```python
from build123d import *

# Parameters (mm, degrees)
BOSS_EXTRUDE1_DEPTH = 6.35
CUT_EXTRUDE18_DEPTH = 10
SKETCH20_R          = 57.15
BOSS_EXTRUDE5_DEPTH = 19.05
CUT_EXTRUDE14_DEPTH = 106.568863781
SKETCH22_R          = 3.175
CUT_EXTRUDE15_DEPTH = 112.672649781
SKETCH24_R          = 5
CUT_EXTRUDE16_DEPTH = 117.574618566
SKETCH25_R          = 2.38125
CUT_EXTRUDE17_DEPTH = 10
CHAMFER2_SIZE       = 2.5
FILLET1_R           = 1.5875
SKETCH28_R          = 30.48
CUT_EXTRUDE19_DEPTH = 105.22344993
CUT_EXTRUDE20_DEPTH = 100.947550226
CUT_EXTRUDE21_DEPTH = 94.849309593


with BuildPart() as part:
    # Sketch1 → Boss-Extrude1 (new body)
    with BuildSketch(Plane(origin=(0, 0, 0), x_dir=(0, 0, -1), z_dir=(1, 0, 0))):
        with BuildLine():
            Line((-30.369265969, -2.595782062), (-25.307721641, -61.813151718))
            ThreePointArc((-25.307721641, -61.813151718), (0, -85.05), (25.307721641, -61.813151718))
            Line((25.307721641, -61.813151718), (30.369265969, -2.595782062))
            ThreePointArc((30.369265969, -2.595782062), (0, 30.48), (-30.369265969, -2.595782062))
        make_face()
        Polygon((4.353205728, 11.960334439), (-11.960334439, 4.353205728), (-4.353205728, -11.960334439), (11.960334439, -4.353205728), align=None, mode=Mode.SUBTRACT)
    extrude(amount=BOSS_EXTRUDE1_DEPTH)

    # Sketch19 → Cut-Extrude18 (cut)
    with BuildSketch(Plane(origin=(6.35, 0, 0), x_dir=(0, 0, -1), z_dir=(1, 0, 0))):
        with BuildLine():
            Line((13.556349186, -39.093650814), (13.556349186, -44.093650814))
            ThreePointArc((13.556349186, -44.093650814), (15.556349186, -46.093650814), (17.556349186, -44.093650814))
            Line((17.556349186, -44.093650814), (17.556349186, -39.093650806))
            ThreePointArc((17.556349186, -39.093650806), (15.556349182, -37.093650814), (13.556349186, -39.093650814))
        make_face()
        with BuildLine():
            Line((-10, -54.65), (-10, -59.65))
            ThreePointArc((-10, -59.65), (0, -69.65), (10, -59.65))
            Line((10, -59.65), (10, -54.65))
            ThreePointArc((10, -54.65), (0, -44.65), (-10, -54.65))
        make_face()
        with BuildLine():
            Line((17.556349186, -75.206349194), (17.556349186, -70.206349186))
            ThreePointArc((17.556349186, -70.206349186), (15.556349186, -68.206349186), (13.556349186, -70.206349186))
            Line((13.556349186, -70.206349186), (13.556349186, -75.206349186))
            ThreePointArc((13.556349186, -75.206349186), (15.556349182, -77.206349186), (17.556349186, -75.206349194))
        make_face()
        with BuildLine():
            Line((-17.556349186, -39.093650806), (-17.556349186, -44.093650814))
            ThreePointArc((-17.556349186, -44.093650814), (-15.556349186, -46.093650814), (-13.556349186, -44.093650814))
            Line((-13.556349186, -44.093650814), (-13.556349186, -39.093650814))
            ThreePointArc((-13.556349186, -39.093650814), (-15.556349182, -37.093650814), (-17.556349186, -39.093650806))
        make_face()
        with BuildLine():
            Line((-13.556349186, -75.206349186), (-13.556349186, -70.206349186))
            ThreePointArc((-13.556349186, -70.206349186), (-15.556349186, -68.206349186), (-17.556349186, -70.206349186))
            Line((-17.556349186, -70.206349186), (-17.556349186, -75.206349194))
            ThreePointArc((-17.556349186, -75.206349194), (-15.556349182, -77.206349186), (-13.556349186, -75.206349186))
        make_face()
    extrude(amount=-CUT_EXTRUDE18_DEPTH, mode=Mode.SUBTRACT)

    # Sketch20 → Boss-Extrude5 (add)
    with BuildSketch(Plane(origin=(6.35, 0, 0), x_dir=(0, 0, -1), z_dir=(1, 0, 0))):
        with Locations(Location((0, 0, 0), (0, 0, 242.654471511))):
            Circle(SKETCH20_R)
    extrude(amount=BOSS_EXTRUDE5_DEPTH)

    # Sketch21 → Cut-Extrude14 (cut, through all)
    with BuildSketch(Plane.ZY):
        Polygon((-19.067760927, 15.897892729), (-24.435012851, 4.387783834), (-10.840396045, -1.951490092), (-5.473144121, 9.558618803), align=None)
        Polygon((-11.960334439, -4.353205728), (-4.353205728, 11.960334439), (11.960334439, 4.353205728), (4.353205728, -11.960334439), align=None)
        Polygon((10.840396045, 1.951490092), (5.473144121, -9.558618803), (19.067760927, -15.897892729), (24.435012851, -4.387783834), align=None)
    extrude(amount=-CUT_EXTRUDE14_DEPTH, mode=Mode.SUBTRACT)

    # Sketch22 → Cut-Extrude15 (cut, through all)
    with BuildSketch(Plane(origin=(0, 5.755054448, 2.683625962), x_dir=(-1, 0, 0), z_dir=(0, -0.9063077870366495, -0.4226182617407005))):
        with Locations(Location((-12.5, -16.5, 0), (0, 0, 90))):
            Circle(SKETCH22_R)
    cut_extrude15 = extrude(amount=-CUT_EXTRUDE15_DEPTH, mode=Mode.SUBTRACT)

    # Sketch24 → Cut-Extrude16 (cut, through all)
    with BuildSketch(Plane(origin=(0, 10.359098006, 4.830526732), x_dir=(-1, 0, 0), z_dir=(0, -0.9063077870366495, -0.4226182617407005))):
        with Locations(Location((-12.5, -16.5, 0), (0, 0, 90))):
            Circle(SKETCH24_R)
    cut_extrude16 = extrude(amount=-CUT_EXTRUDE16_DEPTH, mode=Mode.SUBTRACT)

    # Sketch25 → Cut-Extrude17 (cut)
    with BuildSketch(Plane(origin=(0, -5.755054448, -2.683625962), x_dir=(1, 0, 0), z_dir=(0, 0.9063077870366495, 0.4226182617407006))):
        with Locations(Location((12.5, -16.5, 0), (0, 0, 270))):
            Circle(SKETCH25_R)
    cut_extrude17 = extrude(amount=-CUT_EXTRUDE17_DEPTH, mode=Mode.SUBTRACT)

    # Mirror1: Cut-Extrude15, Cut-Extrude16, Cut-Extrude17 across plane
    add(cut_extrude15.mirror(Plane(origin=(0, 0, 0), x_dir=(1, 0, 0), z_dir=(0, 0.42261826174070105, -0.9063077870366493))), mode=Mode.SUBTRACT)
    add(cut_extrude16.mirror(Plane(origin=(0, 0, 0), x_dir=(1, 0, 0), z_dir=(0, 0.42261826174070105, -0.9063077870366493))), mode=Mode.SUBTRACT)
    add(cut_extrude17.mirror(Plane(origin=(0, 0, 0), x_dir=(1, 0, 0), z_dir=(0, 0.42261826174070105, -0.9063077870366493))), mode=Mode.SUBTRACT)


with BuildPart() as body_2:
    # Mirror2: mirrored copy
    add(part.part.mirror(Plane(origin=(0, 0, 0), x_dir=(0, 0, 1), z_dir=(1, 0, 0))))


with BuildPart() as part_1:
    add(part.part)

    # Chamfer2
    chamfer2_edges = [part_1.edges().sort_by_distance(p)[0] for p in [
        (0, -41.593650814, 13.556349186),
        (0, -37.093650814, 15.556349182),
        (0, -41.59365081, 17.556349186),
        (0, -46.093650814, 15.556349186),
        (0, -41.59365081, -17.556349186),
        (0, -37.093650814, -15.556349182),
        (0, -41.593650814, -13.556349186),
        (0, -46.093650814, -15.556349186),
    ]]
    chamfer(chamfer2_edges, length=CHAMFER2_SIZE)

    # Fillet1
    fillet1_edges = [part_1.edges().sort_by_distance(p)[0] for p in [
        (12.7, 4.387783834, -24.435012851),
        (12.7, 15.897892729, -19.067760927),
        (12.7, -4.387783834, 24.435012851),
        (12.7, -15.897892729, 19.067760927),
        (12.7, 11.960334439, -4.353205728),
        (12.7, 4.353205728, 11.960334439),
        (12.7, -11.960334439, 4.353205728),
        (12.7, -4.353205728, -11.960334439),
    ]]
    fillet(fillet1_edges, radius=FILLET1_R)

    # Sketch28 → Cut-Extrude19 (cut, through all)
    with BuildSketch(Plane(origin=(6.35, 0, 0), x_dir=(0, 0, -1), z_dir=(1, 0, 0))):
        with Locations((0, -54.65)):
            Circle(SKETCH28_R)
    extrude(amount=CUT_EXTRUDE19_DEPTH, mode=Mode.SUBTRACT)

    # Sketch31 → Cut-Revolve1 (revolve, cut)
    with BuildSketch(Plane(origin=(0, 0, 0), x_dir=(1, 0, 0), z_dir=(0, 1, 0)), mode=Mode.PRIVATE) as cut_revolve1_sk:
        Polygon((6.35, -59.952108656), (25.4, -59.952108656), (25.4, -13.97), (6.35, -48.91940088), align=None)
    revolve(cut_revolve1_sk.sketch.rotate(Axis((25.4, 0, 0), (-1, 0, 0)), 2.035690426), axis=Axis((25.4, 0, 0), (-1, 0, 0)), mode=Mode.SUBTRACT)

    # Sketch32 → Cut-Extrude20 (cut, through all)
    with BuildSketch(Plane.ZY.offset(-6.35)):
        with BuildLine():
            Line((30.369265969, -2.595782062), (27.110634253, -40.720035521))
            ThreePointArc((27.110634253, -40.720035521), (0, 48.91940088), (-27.110634253, -40.720035521))
            Line((-27.110634253, -40.720035521), (-30.369265969, -2.595782062))
            ThreePointArc((-30.369265969, -2.595782062), (0, 30.48), (30.369265969, -2.595782062))
        make_face()
    extrude(amount=-CUT_EXTRUDE20_DEPTH, mode=Mode.SUBTRACT)

    # Sketch33 → Cut-Extrude21 (cut, through all)
    with BuildSketch(Plane.ZY):
        with BuildLine():
            Line((29.679571242, -10.664842593), (30.369265969, -2.595782062))
            ThreePointArc((30.369265969, -2.595782062), (28.464776298, 10.898940787), (20.869520673, 22.214713747))
            Line((20.869520673, 22.214713747), (29.679571242, -10.664842593))
        make_face()
    extrude(amount=-CUT_EXTRUDE21_DEPTH, mode=Mode.SUBTRACT)


solid = part_1.part
```
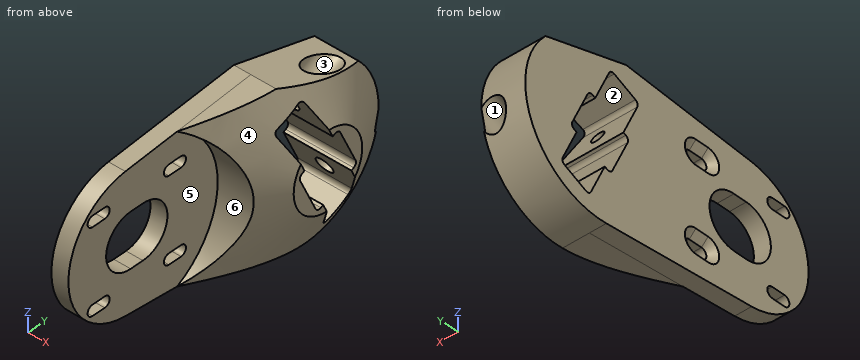
Here's how the part is built. I have some questions about the finished solid (model axes, mm). Face numbers are marked on the shaded views. A direction names the side the tool comes from. Give positions to 0.01 mm unless a question says otherwise; leave off trailing zeros. Loops run counter-clockwise (first coordinate to the right, second up) from the corner with the lowest first, then second, coordinate; pieces in that order, holes last. Notation, with made-up numbers: M 89.5,5.5 L 136.5,5.5 A7 ccw 136.5,13.5 Z; hole C 18.25,17.25 d7. An arc over 180 degrees is marked long. Use one line per item in the form item = value. Start each with the question number.
Q1. If we section it at A-A (y = -52.5): Write out the boundary of the cut face in (x, z).
Q2. If we section it at B-B (y = -73.5): Write out the boundary of the cut face in (x, z), then the cut area to 3 significant figures.
Q3. I need wall thicknesses on line 1 along Y through (x, z) = (3.5, 1); line 2 along Y through (x, z) = (11, 20.5); line 3 along Y through (x, z) = (20.75, 0.5). Which ranges of each line are inside material? Lowest first, please.
Q4. Will these pins go through, and if not, where does the flat tip stop? pin 1 Ø2.5 at (x, y) = (2, -74) entering from +Z; pin 2 Ø2.5 at (x, y) = (3.5, -72.5) entering from -Z; pin 3 Ø3 at (x, y) = (4, -40.5) entering from +Z.
Q5. If we section it at C-C (x = 5.25): State how many separate pieces and enclosed holes the cut face has, then the cut area to 3 significant figures.
Q6. Which directions (+Z, -Z, +X, -X, +Y, -Y) give clear straight access to the entire face, cutting with the end or side of a thin tool? Please do the marked faces 1 and 2.
Q7. Thinking about a two-plate mould opening in Y: for the marked faces 3, 4, 5 and 6, which applies, +Y half, -Y half, draft (parallel to the pull), parting line (faces both ways), or undercut?
Taken from the geometry:
q1.outline = M 0,-26.1 L 6.35,-26.1 L 6.35,-9.77 L 0,-9.77 Z; M 0,9.77 L 6.35,9.77 L 6.35,26.1 L 0,26.1 Z
q2.outline = M 0,-21.29 L 6.35,-21.29 L 6.35,-17.56 L 0,-17.56 Z; M 0,-13.56 L 6.35,-13.56 L 6.35,13.56 L 0,13.56 Z; M 0,17.56 L 6.35,17.56 L 6.35,21.29 L 0,21.29 Z
q2.area = 220 mm^2
q3.line_1 = -85.03 to -69.6, -44.7 to -10.4, 9.46 to 30.46
q3.line_2 = -32.09 to -12.83, -2.55 to -1.7, 16.21 to 22.56
q3.line_3 = -22.5 to -10.16, 9.7 to 22.5
q4.pin_1 = 21.76
q4.pin_2 = -22.6
q4.pin_3 = 27.26
q5.separate_pieces = 1
q5.enclosed_holes = 6
q5.area = 4,470 mm^2
q6.face_1 = none
q6.face_2 = +X, -X
q7.face_3 = undercut
q7.face_4 = parting line
q7.face_5 = draft
q7.face_6 = -Y half
